The model under review builds one solid part; all positions refer to its coordinate system, in mm. Coordinates: 2 decimals unless noted, no trailing zeros. Write each loop counter-clockwise with the first axis right and the second up, starting at its lowest first coordinate (ties: lowest second). Pieces come first, ordered by that corner, then holes.
1) Add section C-C, the plane y = 222. State the section outline as (x, z) points.
2) Mouldability with a two-part tool opening along Z and no side actions: class faces 1 (the flat face through (-44, 304.8, 28)), 2 (the cylindrical face through (32.69, 150.27, 42.63)), 3 (the cylindrical face through (19.812, 150.266, -47.783)) as released by +Z, released by -Z, zero draft, split by the parting line, or undercut.
3) Add section A-A, the plane x = -45. State the section outline as (y, z) points, then the cut area to 3 significant figures.
4) For P1, Ø10, axis at x = 14.5, y = 194, coming from the -Z side; P2, Ø8, axis at x = 39.5, y = 162.5, coming from the -Z side; P3, Ø3, axis at y = 260.35, z = 0, coming from the +X side; P4, Ø2, axis at y = 136, z = -13.5, coming from the +X side, all flat-tipped, find the tip position at first contact; note any pin that passes through.
5) For line 1 (Y direction, x = 53, z = 0); line 2 (X direction, y = 19, z = -11); line 3 (Z direction, x = -17, y = 113.5), list the stretches that pass through material, from the lowest coordinate up.
6) Add section B-B, the plane z = 22. State the section outline as (x, y) points.
from build123d import *

# Parameters (mm, degrees)
SKETCH1_R               = 53.721
SKETCH1_R_2             = 51.7271
BOSS_EXTRUDE1_DEPTH     = 304.8
SKETCH2_R               = 1.7526
BULKHEAD_HOLES_DEPTH    = 127
CIRPATTERN1_COUNT       = 4
CUT_EXTRUDE1_REACH      = 329.617
CUT_EXTRUDE1_END_RADIUS = 51.7271
SKETCH3_R               = 1.7526
CIRPATTERN2_COUNT       = 4


with BuildPart() as part:
    # Sketch1 → Boss-Extrude1 (new body)
    with BuildSketch(Plane(origin=(0, 0, 0), x_dir=(1, 0, 0), z_dir=(0, 1, 0))):
        with Locations(Location((0, 0, 0), (0, 0, 90))):
            Circle(SKETCH1_R)
        with Locations(Location((0, 0, 0), (0, 0, 90))):
            Circle(SKETCH1_R_2, mode=Mode.SUBTRACT)
    extrude(amount=BOSS_EXTRUDE1_DEPTH)

    # Sketch2 → Bulkhead Holes (cut)
    with BuildSketch(Plane.XY):
        with Locations(Location((0, 120.65, 0), (0, 0, 90))):
            Circle(SKETCH2_R)
    bulkhead_holes = extrude(amount=-BULKHEAD_HOLES_DEPTH, mode=Mode.SUBTRACT)

    # CirPattern1: Bulkhead Holes ×4 about axis
    cirpattern1_axis = Axis((0, 304.8, 0), (0, -1, 0))
    for i in range(1, CIRPATTERN1_COUNT):
        add(bulkhead_holes.rotate(cirpattern1_axis, i * 360 / CIRPATTERN1_COUNT), mode=Mode.SUBTRACT)

    # Cut-Extrude1: up to this cylinder (the profile starts outside it)
    cut_extrude1_end = Plane(origin=(0, 260.35, 0), z_dir=(0, -1, 0)) * Cylinder(CUT_EXTRUDE1_END_RADIUS, 763.6882, mode=Mode.PRIVATE)
    # Sketch3 → Cut-Extrude1 (cut, up to the surface)
    with BuildSketch(Plane(origin=(53.721, 0, 0), x_dir=(0, 0, -1), z_dir=(1, 0, 0)), mode=Mode.PRIVATE) as cut_extrude1_sk1:
        with Locations((0, 260.35)):
            Circle(SKETCH3_R)
    cut_extrude1_tool1 = extrude(cut_extrude1_sk1.sketch, amount=-CUT_EXTRUDE1_REACH, mode=Mode.PRIVATE) - cut_extrude1_end
    cut_extrude1 = cut_extrude1_tool1.solids().sort_by_distance((53.721, 260.35, 0))[0]
    add(cut_extrude1, mode=Mode.SUBTRACT)

    # CirPattern2: Cut-Extrude1 ×4 about axis
    cirpattern2_axis = Axis((0, 304.8, 0), (0, -1, 0))
    for i in range(1, CIRPATTERN2_COUNT):
        add(cut_extrude1.rotate(cirpattern2_axis, i * 360 / CIRPATTERN2_COUNT), mode=Mode.SUBTRACT)


solid = part.part
Geometry results:
1. outline: circle Ø107.44 at (0, 0); hole circle Ø103.45 at (0, 0)
2. face 1: zero draft
2. face 2: split by the parting line
2. face 3: undercut
3. outline: (0, -29.34) - (304.8, -29.34) - (304.8, -25.51) - (0, -25.51) - close; (0, 25.51) - (304.8, 25.51) - (304.8, 29.34) - (0, 29.34) - close
3. area: 2,340 mm2
4. P1: stops at z = -52.87
4. P2: stops at z = -40.32
4. P3: passes through
4. P4: stops at x = 52.25
5. line 1: y = 0 to 118.9, 122.4 to 258.6, 262.1 to 304.8
5. line 2: x = -52.58 to -50.54, 50.54 to 52.58
5. line 3: z = -50.96 to -48.85, 48.85 to 50.96
6. outline: (-49.01, 0) - (-46.82, 0) - (-46.82, 304.8) - (-49.01, 304.8) - close; (46.82, 0) - (49.01, 0) - (49.01, 304.8) - (46.82, 304.8) - close
